```python
from build123d import *

# Parameters (mm, degrees)
BOSS_EXTRUDE1_DEPTH = 1.8
SKETCH2_W           = 6
SKETCH2_H           = 12
BOSS_EXTRUDE2_DEPTH = 0.75
SKETCH7_W           = 1.65
SKETCH7_H           = 3.8
CUT_EXTRUDE2_DEPTH  = 0.4
SKETCH9_R           = 0.4
CUT_EXTRUDE4_DEPTH  = 0.2
BOSS_EXTRUDE3_DEPTH = 2.7
SKETCH11_W          = 2.7
SKETCH11_H          = 1.5
CUT_EXTRUDE5_DEPTH  = 1.5


with BuildPart() as part:
    # Sketch1 → Boss-Extrude1 (new body)
    with BuildSketch(Plane(origin=(0, 0, 0), x_dir=(1, 0, 0), z_dir=(0, 1, 0))):
        Polygon((-1.4, 3), (-1.4, 0), (-1.975, 0), (-1.975, -1.5), (1.975, -1.5), (1.975, 0), (1.4, 0), (1.4, 3), (3, 3), (3, -9), (-3, -9), (-3, 3), align=None)
    extrude(amount=BOSS_EXTRUDE1_DEPTH)

    # Sketch2 → Boss-Extrude2 (add)
    with BuildSketch(Plane.XZ):
        with Locations((0, 3)):
            Rectangle(SKETCH2_W, SKETCH2_H)
    extrude(amount=BOSS_EXTRUDE2_DEPTH)

    # Sketch7 → Cut-Extrude2 (cut)
    with BuildSketch(Plane(origin=(0, 1.8, 0), x_dir=(1, 0, 0), z_dir=(0, 1, 0))):
        with Locations((-2.175, -4.5)):
            Rectangle(SKETCH7_W, SKETCH7_H)
        with Locations((2.175, -4.5)):
            Rectangle(SKETCH7_W, SKETCH7_H)
    extrude(amount=-CUT_EXTRUDE2_DEPTH, mode=Mode.SUBTRACT)

    # Sketch9 → Cut-Extrude4 (cut)
    with BuildSketch(Plane(origin=(3, 0, 0), x_dir=(0, 0, -1), z_dir=(1, 0, 0))):
        with Locations((1.9, 0.8)):
            Circle(SKETCH9_R)
    cut_extrude4 = extrude(amount=-CUT_EXTRUDE4_DEPTH, mode=Mode.SUBTRACT)

    # Mirror1: Cut-Extrude4 across plane
    add(cut_extrude4.mirror(Plane(origin=(0, 0, 0), x_dir=(0, 0, 1), z_dir=(1, 0, 0))), mode=Mode.SUBTRACT)

    # Sketch10 → Boss-Extrude3 (add)
    with BuildSketch(Plane(origin=(0, 1.8, 0), x_dir=(1, 0, 0), z_dir=(0, 1, 0))):
        Polygon((-1.35, -6.4), (-1.35, -9), (1.35, -9), (1.35, -6.4), (1.35, -2.6), (1.35, -1.5), (-1.35, -1.5), (-1.35, -2.6), align=None)
    extrude(amount=BOSS_EXTRUDE3_DEPTH)

    # Sketch11 → Cut-Extrude5 (cut)
    with BuildSketch(Plane(origin=(0, 4.5, 0), x_dir=(1, 0, 0), z_dir=(0, 1, 0))):
        with Locations((0, -4.5)):
            Rectangle(SKETCH11_W, SKETCH11_H)
    extrude(amount=-CUT_EXTRUDE5_DEPTH, mode=Mode.SUBTRACT)


solid = part.part
```
Model file for the job. Use its own axes, mm. A direction names the side the tool comes from. Round coordinates to 2 decimals unless told otherwise and drop trailing zeros. Write each loop counter-clockwise with the first axis right and the second up, starting at its lowest first coordinate (ties: lowest second). Pieces come first, ordered by that corner, then holes. Notation, with made-up numbers: (4, -24.5) -> (16, -24.5) arc R14 ccw to (16, -20.5) -> close; hole circle Ø2 at (18, 32). An arc over 180 degrees is marked (long way). Answer as CSV lines item,"result".
1. Mould opens along X. For faces 5 (the face through (0, 2, 1.5)), 6 (the face through (-3, 1, 3)), 7 (the face through (0, 4, 5.25)) say: +X half, -X half, draft (parallel to the pull), parting line (faces both ways), or undercut.
Resolved:
face 5,"undercut"
face 6,"-X half"
face 7,"draft"
2. Slice it at A-A, the plane y = 3.8. List the corners of the cut face in (x, z).
Resolved:
outline,"(-1.35, 1.5) -> (1.35, 1.5) -> (1.35, 3.75) -> (-1.35, 3.75) -> close; (-1.35, 5.25) -> (1.35, 5.25) -> (1.35, 9) -> (-1.35, 9) -> close"
3. Slice it at D-D, the plane y = 0.8. List the corners of the cut face in (x, z) (3 decimals).
Resolved:
outline,"(-3, -3) -> (-1.4, -3) -> (-1.4, 0) -> (-1.975, 0) -> (-1.975, 1.5) -> (1.975, 1.5) -> (1.975, 0) -> (1.4, 0) -> (1.4, -3) -> (3, -3) -> (3, -2.3) -> (2.8, -2.3) -> (2.8, -1.5) -> (3, -1.5) -> (3, 9) -> (-3, 9) -> (-3, -1.5) -> (-2.8, -1.5) -> (-2.8, -2.3) -> (-3, -2.3) -> close"
4. Tool access for faces 1 (the face through (1.975, 1, 1)), 2 (the face through (0, 4, 3.75)), 3 (the face through (-2, 1.8, 8)), 4 (the face through (-2, 1.4, 4)): list every direction of +Z, -Z, +X, -X, +Y, -Y with a clear straight run to the whole face (end or side of a thin tool).
Resolved:
face 1,"+Y"
face 2,"+X, -X, +Y"
face 3,"+Z, -Z, -X, +Y"
face 4,"-X, +Y"
5. Slice it at C-C, the plane x = -1.15. List the corners of the cut face in (y, z), plus the area to 3 significant figures.
Resolved:
outline,"(-0.75, -3) -> (0, -3) -> (0, 1.5) -> (4.5, 1.5) -> (4.5, 3.75) -> (3, 3.75) -> (3, 5.25) -> (4.5, 5.25) -> (4.5, 9) -> (-0.75, 9) -> close"
area,"40.5 mm²"
6. Slice it at B-B, the plane z = 4.5. List the corners of the cut face in (x, y).
Resolved:
outline,"(-3, -0.75) -> (3, -0.75) -> (3, 1.4) -> (1.35, 1.4) -> (1.35, 3) -> (-1.35, 3) -> (-1.35, 1.4) -> (-3, 1.4) -> close"
7. Drill centre lines: line 1 (Y direction, x = 2.9, z = -1.9); line 2 (Z direction, x = 1.15, y = 3.4); line 3 (Z direction, x = 1, y = 1.4). Where is each one in solid material? Low to high.
Resolved:
line 1,"-0.75 to 0.4, 1.2 to 1.8"
line 2,"1.5 to 3.75, 5.25 to 9"
line 3,"1.5 to 9"
8. Pin check, flat tips, straight feed: pin 1 Ø1.6 at (x, y) = (0.5, 3.5) entering from -Z; pin 2 Ø1.6 at (y, z) = (3, 5.5) entering from +X; pin 3 Ø0.5 at (x, z) = (2.5, 5) entering from +Y. Stop position of each tip, or through.
Resolved:
pin 1,"z = 1.5"
pin 2,"x = 1.35"
pin 3,"y = 1.4"
